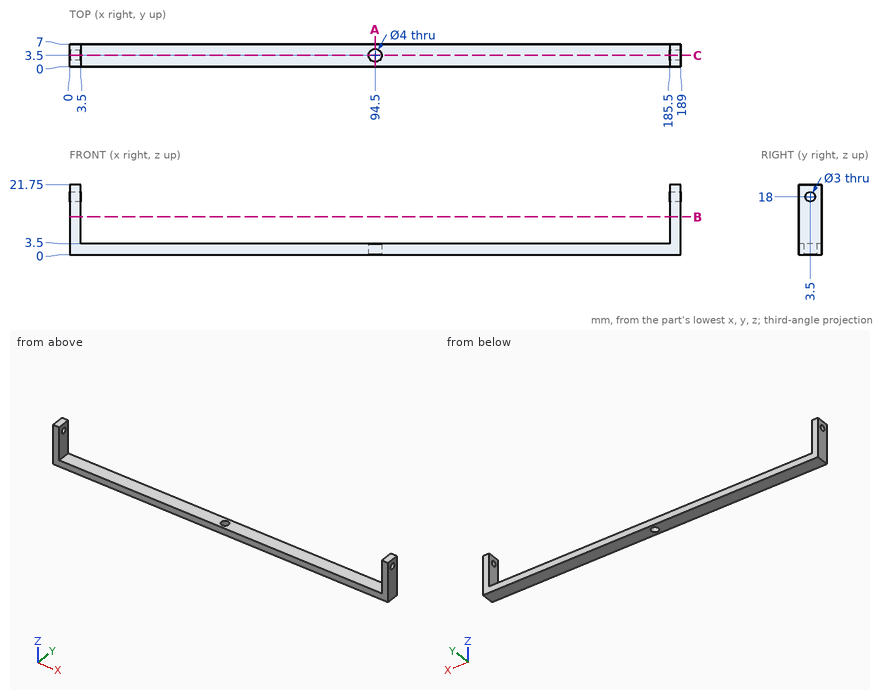
Study the drawing (mm; zero at the part's minimum x, y, z) and answer. Give positions to 0.01 mm unless a question says otherwise; leave off trailing zeros. Order: outer loops, then holes, each group sorted by start corner. A loop starts at its lowest first (then second) coordinate and runs counter-clockwise, first axis right, second up.
1) Find section A-A on x = 94.5. Write down the section's boundary in (y, z), then the cut area to 3 significant figures.
Reported:
outline: (0, 0) - (1.5, 0) - (1.5, 3.5) - (0, 3.5) - close; (5.5, 0) - (7, 0) - (7, 3.5) - (5.5, 3.5) - close
area: 10.5 mm2
2) Find section B-B on z = 11.75. Write down the section's boundary in (x, y), then the cut area to 3 significant figures.
Reported:
outline: (0, 0) - (3.5, 0) - (3.5, 7) - (0, 7) - close; (185.5, 0) - (189, 0) - (189, 7) - (185.5, 7) - close
area: 49.0 mm2
3) Find section C-C on y = 3.5. Write down the section's boundary in (x, z).
Reported:
outline: (0, 0) - (92.5, 0) - (92.5, 3.5) - (3.5, 3.5) - (3.5, 16.5) - (0, 16.5) - close; (0, 19.5) - (3.5, 19.5) - (3.5, 21.75) - (0, 21.75) - close; (96.5, 0) - (189, 0) - (189, 16.5) - (185.5, 16.5) - (185.5, 3.5) - (96.5, 3.5) - close; (185.5, 19.5) - (189, 19.5) - (189, 21.75) - (185.5, 21.75) - close
4) Given P1, Ø2.5, axis at y = 3.5, z = 18, coming from the -X side; P2, Ø1, axis at x = 123, y = 5.5, coming from the +Z side, each flat-ended and moving along its own axis, determine where each tip first touches the part or whether it passes through.
Reported:
P1: passes through
P2: stops at z = 3.5
5) Consider line 1 along X through (y, z) = (6, 18); line 2 along Y through (x, z) = (1.95, 18); line 3 along Z through (x, y) = (57, 5.75). Determine where each line is inside the solid, lowest interval first.
Reported:
line 1: x = 0 to 3.5, 185.5 to 189
line 2: y = 0 to 2, 5 to 7
line 3: z = 0 to 3.5
